from build123d import *

# Parameters (mm, degrees)
BOSS_EXTRUDE1_DEPTH      = 48.26
FILLET1_R                = 2.5399999999999996
BOSS_EXTRUDE2_START      = -48.26
BOSS_EXTRUDE2_DEPTH      = 2.5399999999999996
BOSS_EXTRUDE3_START      = 48.26
BOSS_EXTRUDE3_DEPTH      = 2.5399999999999996
CUT_EXTRUDE2_START       = -29.21
SKETCH4_R                = 6.349999999999995
CUT_EXTRUDE2_DEPTH       = 2.54
FILLET2_R                = 2.5399999999999996
M4_CLEARANCE_HOLE1_D     = 4.5
M4_CLEARANCE_HOLE1_DEPTH = 2.54


with BuildPart() as part:
    # Sketch1 → Boss-Extrude1 (new, symmetric)
    with BuildSketch(Plane(origin=(0, 0, 0), x_dir=(0, 0, -1), z_dir=(1, 0, 0))):
        Polygon((31.75, -7.8e-16), (-31.75, -8.55e-15), (-31.75, 38.099999999999994), (-29.21, 38.099999999999994), (-29.209999999999997, 2.539999999999991), (-19.049999999999997, 2.539999999999991), (-19.049999999999997, 1.2699999999999922), (-6.350000000000001, 1.2699999999999922), (-6.35, 2.5399999999999943), (6.35, 2.539999999999996), (6.350000000000001, 1.2699999999999938), (19.049999999999997, 1.2699999999999971), (19.049999999999997, 2.539999999999996), (29.209999999999997, 2.539999999999998), (29.209999999999994, 38.1), (31.749999999999986, 38.1), align=None)
    extrude(amount=BOSS_EXTRUDE1_DEPTH, both=True)

    # Fillet1
    fillet1_edges = [part.edges().sort_by_distance(p)[0] for p in [
        (0, -8.55e-15, 31.75),
        (0, -7.8e-16, -31.75),
        (0, 2.539999999999998, -29.209999999999997),
        (0, 2.539999999999991, 29.209999999999997),
    ]]
    fillet(fillet1_edges, radius=FILLET1_R)

    # Sketch3 → Boss-Extrude2 (add)
    with BuildSketch(Plane(origin=(0, 0, 0), x_dir=(0, 0, -1), z_dir=(1, 0, 0)).offset(BOSS_EXTRUDE2_START)):
        with BuildLine():
            Line((0, 38.099999999999994), (-31.75, 38.099999999999994))
            Line((-31.75, 38.099999999999994), (-31.75, 2.539999999999992))
            ThreePointArc((-31.75, 2.5399999999999934), (-31.00605122421383, 0.7439487757861607), (-29.209999999999997, -7.55e-15))
            Line((-29.209999999999997, -7.81e-15), (0, -4.23e-15))
            Line((0, 0), (1.56e-15, 38.099999999999994))
        make_face()
        with BuildLine():
            Line((31.75, 38.1), (0, 38.099999999999994))
            Line((1.56e-15, 38.099999999999994), (0, 0))
            Line((0, -4.23e-15), (29.210000000000004, -6.5e-16))
            ThreePointArc((29.210000000000004, -2.22e-15), (31.00605122421384, 0.7439487757861647), (31.750000000000014, 2.540000000000001))
            Line((31.750000000000014, 2.539999999999999), (31.75, 38.1))
        make_face()
    extrude(amount=BOSS_EXTRUDE2_DEPTH)

    # Sketch3<3> → Boss-Extrude3 (add)
    with BuildSketch(Plane(origin=(0, 0, 0), x_dir=(0, 0, -1), z_dir=(1, 0, 0)).offset(BOSS_EXTRUDE3_START)):
        with BuildLine():
            Line((31.75, 38.1), (0, 38.099999999999994))
            Line((1.56e-15, 38.099999999999994), (0, 0))
            Line((0, -4.23e-15), (29.210000000000004, -6.5e-16))
            ThreePointArc((29.210000000000004, -2.22e-15), (31.00605122421384, 0.7439487757861647), (31.750000000000014, 2.540000000000001))
            Line((31.750000000000014, 2.539999999999999), (31.75, 38.1))
        make_face()
        with BuildLine():
            Line((0, 38.099999999999994), (-31.75, 38.099999999999994))
            Line((-31.75, 38.099999999999994), (-31.75, 2.539999999999992))
            ThreePointArc((-31.75, 2.5399999999999934), (-31.00605122421383, 0.7439487757861607), (-29.209999999999997, -7.55e-15))
            Line((-29.209999999999997, -7.81e-15), (0, -4.23e-15))
            Line((0, 0), (1.56e-15, 38.099999999999994))
        make_face()
    extrude(amount=BOSS_EXTRUDE3_DEPTH)

    # Sketch4 → Cut-Extrude2 (cut)
    with BuildSketch(Plane.XY.offset(CUT_EXTRUDE2_START)):
        with Locations(Location((40.63999999999999, 10.159999999999991, 0), (0, 0, 306.869897646))):
            Circle(SKETCH4_R)
    extrude(amount=-CUT_EXTRUDE2_DEPTH, mode=Mode.SUBTRACT)

    # Fillet2
    fillet2_edges = [part.edges().sort_by_distance(p)[0] for p in [
        (50.8, 20.319999999999993, 31.75),
        (50.8, 0.7439487757861605, 31.00605122421383),
        (50.8, -4.78e-15, -3.55e-15),
        (50.8, 0.7439487757861649, -31.00605122421384),
        (50.8, 20.32, -31.750000000000007),
        (-48.26, 20.32, -31.749999999999993),
        (-48.26, -4.67e-15, 0),
        (-48.26, 20.319999999999993, 31.75),
        (-48.26, 0.7439487757861611, 31.00605122421383),
        (-48.26, 0.7439487757861682, -31.00605122421383),
    ]]
    fillet(fillet2_edges, radius=FILLET2_R)

    # M4 Clearance Hole1
    with Locations(Plane.XY.offset(-29.209999999999997)):
        with Locations((-38.1, 30.48), (40.64, 30.48), (-38.1, 10.16)):
            Hole(M4_CLEARANCE_HOLE1_D / 2, depth=M4_CLEARANCE_HOLE1_DEPTH)


solid = part.part
Verification items for the finished model (mm, model axes). A direction names the side the tool comes from. Coordinates: 2 decimals unless noted, no trailing zeros. Order: outer loops, then holes, each group sorted by start corner. A loop starts at its lowest first (then second) coordinate and runs counter-clockwise, first axis right, second up.
1. Sectioned sample at A-A, the plane y = 30.48. Record the cut outline in (x, z).
Results found:
outline: (-48.26, -29.21) arc R2.54 ccw to (-45.72, -31.75) - (-40.35, -31.75) - (-40.35, -29.21) - (-45.72, -29.21) - (-45.72, 29.21) - (48.26, 29.21) - (48.26, -29.21) - (42.89, -29.21) - (42.89, -31.75) - (48.26, -31.75) arc R2.54 ccw to (50.8, -29.21) - (50.8, 29.21) arc R2.54 ccw to (48.26, 31.75) - (-45.72, 31.75) arc R2.54 ccw to (-48.26, 29.21) - close; (-35.85, -31.75) - (38.39, -31.75) - (38.39, -29.21) - (-35.85, -29.21) - close
2. Release check for a two-part mould opening along Z. For faces 1 (the face through (48.26, 20, 0)), 2 (the face through (1, 21, 31.75)), 3 (the face through (1, 38.1, -31)) record: +Z half, -Z half, draft (parallel to the pull), parting line (faces both ways), or undercut.
Results found:
face 1: undercut
face 2: +Z half
face 3: draft
3. Sectioned sample at C-C, the plane x = 3. Record the cut outline in (y, z).
Results found:
outline: (0, -29.21) arc R2.54 ccw to (2.54, -31.75) - (38.1, -31.75) - (38.1, -29.21) - (5.08, -29.21) arc R2.54 cw to (2.54, -26.67) - (2.54, -19.05) - (1.27, -19.05) - (1.27, -6.35) - (2.54, -6.35) - (2.54, 6.35) - (1.27, 6.35) - (1.27, 19.05) - (2.54, 19.05) - (2.54, 26.67) arc R2.54 cw to (5.08, 29.21) - (38.1, 29.21) - (38.1, 31.75) - (2.54, 31.75) arc R2.54 ccw to (0, 29.21) - close
4. Go/stop test with flat-tipped pins: pin 1 Ø10 at (x, z) = (-20, -14.5) entering from +Y; pin 2 Ø4 at (x, z) = (-15.5, 14) entering from +Y; pin 3 Ø0.6 at (x, y) = (17.5, 1.5) entering from +Z. Record where each tip stops, or that it passes through.
Results found:
pin 1: stops at y = 2.54
pin 2: stops at y = 1.27
pin 3: stops at z = 31.64
5. Sectioned sample at B-B, the plane x = -38.1. Record the cut outline in (y, z).
Results found:
outline: (0, -29.21) arc R2.54 ccw to (2.54, -31.75) - (7.91, -31.75) - (7.91, -29.21) - (5.08, -29.21) arc R2.54 cw to (2.54, -26.67) - (2.54, -19.05) - (1.27, -19.05) - (1.27, -6.35) - (2.54, -6.35) - (2.54, 6.35) - (1.27, 6.35) - (1.27, 19.05) - (2.54, 19.05) - (2.54, 26.67) arc R2.54 cw to (5.08, 29.21) - (38.1, 29.21) - (38.1, 31.75) - (2.54, 31.75) arc R2.54 ccw to (0, 29.21) - close; (12.41, -31.75) - (28.23, -31.75) - (28.23, -29.21) - (12.41, -29.21) - close; (32.73, -31.75) - (38.1, -31.75) - (38.1, -29.21) - (32.73, -29.21) - close
6. Sectioned sample at D-D, the plane y = 35.5. Record the cut outline in (x, z), and give its area (3 significant figures).
Results found:
outline: (-48.26, -29.21) arc R2.54 ccw to (-45.72, -31.75) - (48.26, -31.75) arc R2.54 ccw to (50.8, -29.21) - (50.8, 29.21) arc R2.54 ccw to (48.26, 31.75) - (-45.72, 31.75) arc R2.54 ccw to (-48.26, 29.21) - close; hole (-45.72, -29.21) - (48.26, -29.21) - (48.26, 29.21) - (-45.72, 29.21) - close
area: 794 mm2
7. Scan lines: line 1 (Z direction, x = 28.5, y = 13.5); line 2 (X direction, y = 14.5, z = 25); line 3 (X direction, y = 10, z = -30). Record each from-to range of solid material in increasing order.
Results found:
line 1: z = -31.75 to -29.21, 29.21 to 31.75
line 2: x = -48.26 to -45.72, 48.26 to 50.8
line 3: x = -48.13 to -40.34, -35.86 to 34.29, 46.99 to 50.67
8. Set-up check for faces 4 (the face through (1, 0, 0)), 5 (the face through (-35.852, 10.259, -30.498)), 6 (the face through (2, 2.54, 0)): record each of +Z, -Z, +X, -X, +Y, -Y from which the full face is reachable in a straight line by a thin tool's end or side.
Results found:
face 4: +Z, -Z, +X, -X, -Y
face 5: -Z
face 6: +Y
